Autodesk Inventor part; units mm, degrees
ref_plane "YZ Plane" through (0, 0, 0) normal (1, 0, 0) x (0, 1, 0)
ref_plane "XZ Plane" through (0, 0, 0) normal (0, 1, 0) x (-1, 0, 0)
ref_plane "XY Plane" through (0, 0, 0) normal (0, 0, 1) x (1, 0, 0)
sketch "Sketch1" plane through (0, 0, 0) normal (0, 0, 1) x (1, 0, 0)
  line L0 (-4, -8) -> (22.5, -5)
  line L1 (26, -1.5) -> (26, 1.5)
  line L2 (22.5, 5) -> (-4, 8)
  line L3 (-8, 4) -> (-8, -4)
  line L4 (-4, 8) -> (-8, 4)
  line L5 (-8, -4) -> (-4, -8)
  line L6 (22.5, -5) -> (26, -1.5)
  line L7 (26, 1.5) -> (22.5, 5)
  circle A0 centre (0, 0) radius 2.75
  circle A1 centre (20, 0) radius 2.25
  circle A2 centre (0, 0) radius 5 construction
  circle A3 centre (20, 0) radius 4.5 construction
  point P0 (-8, 0)
  point P1 (26, 0)
  dimension "d9" = 8
  dimension "d10" = 20
  dimension "d11" = 4.5
  dimension "d12" = 5.5
  dimension "d13" = 6
  dimension "d16" = 10
  dimension "d17" = 9
  dimension "d18" = 8
  dimension "d19" = 4
  dimension "d20" = 4
  dimension "d21" = 4
  dimension "d22" = 10
  dimension "d23" = 3
extrude "Extrusion1" add sketch "Sketch1" along normal blind 6
sketch "Sketch2" plane through (0, 0, 6) normal (0, 0, 1) x (1, 0, 0)
  circle A0 centre (0, 0) radius 2.75
  line L0 (-8, 4) -> (-8, -4)
  line L1 (4.6188, 0) -> (2.3094, -4)
  line L2 (2.3094, -4) -> (-2.3094, -4)
  line L3 (-2.3094, -4) -> (-4.6188, 0)
  line L4 (-4.6188, 0) -> (-2.3094, 4)
  line L5 (-2.3094, 4) -> (2.3094, 4)
  line L6 (2.3094, 4) -> (4.6188, 0)
  dimension "d24" = 8
extrude "Extrusion2" cut sketch "Sketch2" against normal through all
properties part number "y_carriage_nut_holder_b"
Work out the finished part from the listing and answer in its coordinate system (mm). A direction names the side the tool comes from. Round coordinates to 2 decimals unless told otherwise and drop trailing zeros. Order: outer loops, then holes, each group sorted by start corner. A loop starts at its lowest first (then second) coordinate and runs counter-clockwise, first axis right, second up.
Q1. A tool of negligible diameter and unlimited length cuts with its end or side. For faces 4 (the flat face through (0, 4, 3)), 5 (the flat face through (9.06, -6.52, 2.96)), from which of +Z, -Z, +X, -X, +Y, -Y can it reach the whole face along a straight path? Write none if from no direction.
Solution:
face 4: +Z, -Z
face 5: +Z, -Z, +X, -Y
Q2. A cutting plane is placed at B-B, the plane x = 20. Determine the outline of the cut face in (y, z).
Solution:
outline: (-5.28, 0) - (-2.25, 0) - (-2.25, 6) - (-5.28, 6) - close; (2.25, 0) - (5.28, 0) - (5.28, 6) - (2.25, 6) - close
Q3. Find the intervals of material crossed by line 1 along X through (y, z) = (-1.25, 4.2); line 2 along Y through (x, z) = (1.5, 4.35); line 3 along Y through (x, z) = (20, 4.65), in increasing order.
Solution:
line 1: x = -8 to -3.9, 3.9 to 18.13, 21.87 to 26
line 2: y = -7.38 to -4, 4 to 7.38
line 3: y = -5.28 to -2.25, 2.25 to 5.28
Q4. A cutting plane is placed at A-A, the plane z = 1.1. Determine the outline of the cut face in (x, y).
Solution:
outline: (-8, -4) - (-4, -8) - (22.5, -5) - (26, -1.5) - (26, 1.5) - (22.5, 5) - (-4, 8) - (-8, 4) - close; hole (-4.62, 0) - (-2.31, -4) - (2.31, -4) - (4.62, 0) - (2.31, 4) - (-2.31, 4) - close; hole circle Ø4.5 at (20, 0)
Q5. A cutting plane is placed at D-D, the plane x = 8.5. Determine the outline of the cut face in (y, z), then the cut area to 3 significant figures.
Solution:
outline: (-6.58, 0) - (6.58, 0) - (6.58, 6) - (-6.58, 6) - close
area: 79.0 mm2
Q6. Given pin 1 Ø3 at (x, z) = (20, 2.5) entering from +Y; pin 2 Ø2.5 at (x, z) = (-0.5, 1.5) entering from -Y; pin 3 Ø2.5 at (x, z) = (0, 2.5) entering from +Y, each flat-ended and moving along its own axis, determine where each tip first touches the part or whether it passes through.
Solution:
pin 1: stops at y = 5.45
pin 2: stops at y = -7.75
pin 3: stops at y = 7.69
Q7. The mould has two halves that part along X. Classify faces 1 (the flat face through (24.3, 3.2, 3)), 2 (the flat face through (0, -4, 3)), 3 (the flat face through (-8, 0, 3)): pulls with the +X half, pulls with the -X half, needs draft (parallel to the pull), parting line crosses it, or undercut.
Solution:
face 1: pulls with the +X half
face 2: undercut
face 3: pulls with the -X half
Q8. A cutting plane is placed at C-C, the plane y = -6.5. Determine the outline of the cut face in (x, z), then the cut area to 3 significant figures.
Solution:
outline: (-5.5, 0) - (9.25, 0) - (9.25, 6) - (-5.5, 6) - close
area: 88.5 mm2
